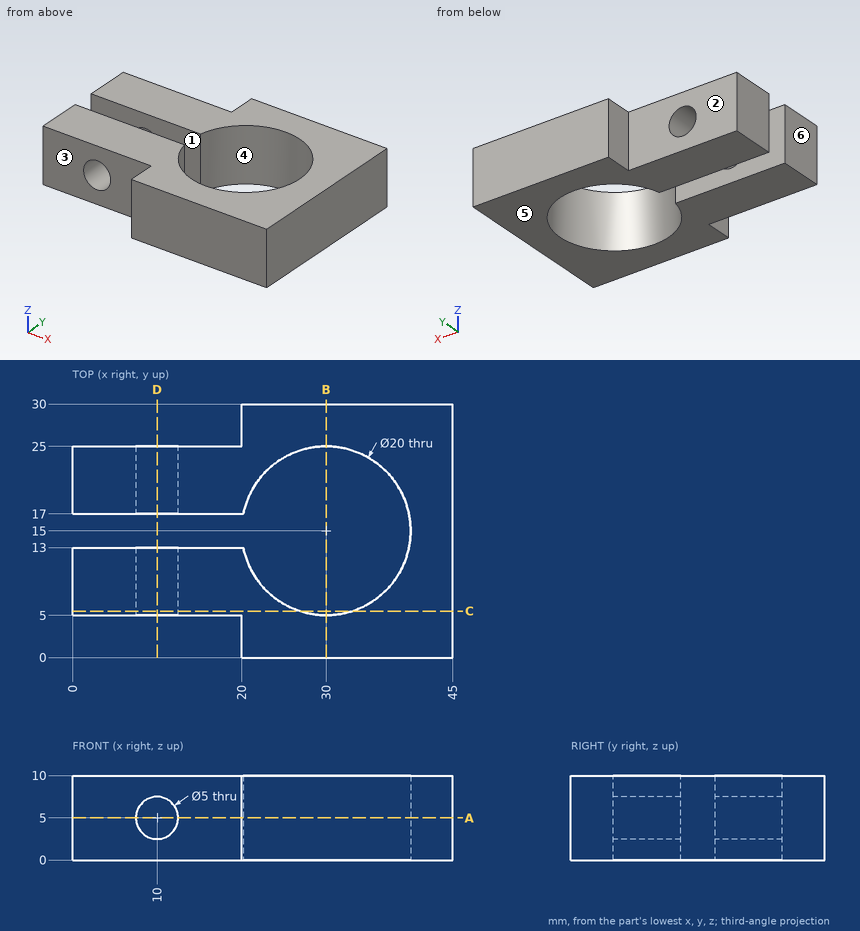
Drawing for the job (mm, zero at the part's lowest x, y, z). A direction names the side the tool comes from. Round coordinates to 2 decimals unless told otherwise and drop trailing zeros. Loops run counter-clockwise (first coordinate to the right, second up) from the corner with the lowest first, then second, coordinate; pieces in that order, holes last. Notation, with made-up numbers: (-6, 68.5) - (28, 68.5) arc R14 ccw to (28, 86.5) - close; hole circle Ø5 at (3.25, 50.25). An arc over 180 degrees is marked (long way). Return JSON: item names as keys, results as strings. Group by question number.
Q1. Flat gauge pins, fed straight in: pin 1 Ø2 at (y, z) = (13.5, 7) entering from -X; pin 2 Ø3 at (x, z) = (10, 5) entering from +Y; pin 3 Ø1.5 at (y, z) = (26.5, 2.5) entering from -X; pin 4 Ø3 at (x, z) = (17, 8) entering from +Y. Where does each tip first touch, or does it go through?
Q2. Band-saw the part on C-C on y = 5.5. Give the cut face in (x, z).
Q3. Tool access for the marked faces 1, 2 and 3: list every direction of +Z, -Z, +X, -X, +Y, -Y with a clear straight run to the whole face (end or side of a thin tool).
Q4. Band-saw the part on D-D on x = 10. Give the cut face in (y, z), plus the area to 3 significant figures.
Q5. Band-saw the part on B-B on x = 30. Give the cut face in (y, z).
Q6. Two-plate mould, pull along X, no slides. Class the marked faces 4, 5 and 6: +X half, -X half, draft (parallel to the pull), parting line (faces both ways), or undercut.
Q7. Band-saw the part on A-A on z = 5. Give the cut face in (x, y).
Q8. Drill centre lines: line 1 along Y through (x, z) = (13, 6); line 2 along Z through (x, y) = (10, 22); line 3 along X through (y, z) = (17.25, 2.75). Where is each one in solid material? Low to high. Write a range as [from, to].
Solutions:
{
 "1": {"pin 1": "stops at x = 0", "pin 2": "passes through", "pin 3": "stops at x = 20", "pin 4": "stops at y = 25"},
 "2": {"outline": "(0, 0) - (26.88, 0) - (26.88, 10) - (0, 10) - close; (33.12, 0) - (45, 0) - (45, 10) - (33.12, 10) - close; hole circle Ø5 at (10, 5)"},
 "3": {"face 1": "+Z, -Z, -X", "face 2": "+Z, -Z, -X, +Y", "face 3": "+Z, -Z, -X, -Y"},
 "4": {"outline": "(5, 0) - (13, 0) - (13, 2.5) - (5, 2.5) - close; (5, 7.5) - (13, 7.5) - (13, 10) - (5, 10) - close; (17, 0) - (25, 0) - (25, 2.5) - (17, 2.5) - close; (17, 7.5) - (25, 7.5) - (25, 10) - (17, 10) - close", "area": "80.0 mm^2"},
 "5": {"outline": "(0, 0) - (5, 0) - (5, 10) - (0, 10) - close; (25, 0) - (30, 0) - (30, 10) - (25, 10) - close"},
 "6": {"face 4": "undercut", "face 5": "draft", "face 6": "-X half"},
 "7": {"outline": "(0, 5) - (7.5, 5) - (7.5, 13) - (0, 13) - close; (0, 17) - (7.5, 17) - (7.5, 25) - (0, 25) - close; (12.5, 5) - (20, 5) - (20, 0) - (45, 0) - (45, 30) - (20, 30) - (20, 25) - (12.5, 25) - (12.5, 17) - (20.2, 17) arc R10 cw (long way) to (20.2, 13) - (12.5, 13) - close"},
 "8": {"line 1": "y = [5, 13], [17, 25]", "line 2": "z = [0, 2.5], [7.5, 10]", "line 3": "x = [0, 8.91], [11.09, 20.26], [39.74, 45]"}
}
